For this review, take the finished solid that the model builds, in its own axes (mm). Face numbers are marked on the shaded views. Coordinates: 2 decimals unless noted, no trailing zeros. Order: outer loops, then holes, each group sorted by start corner. A loop starts at its lowest first (then second) coordinate and runs counter-clockwise, first axis right, second up. Notation, with made-up numbers: (56.25, 40.5) -> (115.25, 40.5) arc R23 cw to (115.25, 52.5) -> close; hole circle Ø2 at (-34.5, 1.25). An arc over 180 degrees is marked (long way). Answer as a JSON object with one key per item and string values. Group by question number.
1) Draft analysis for pull direction X (two halves, no side actions). For the marked faces 1, 2 and 3, state which applies: +X half, -X half, draft (parallel to the pull), parting line (faces both ways), or undercut.
2) Add section B-B, the plane x = 0. Write out the cut boundary in (y, z).
3) For pin 1 (8 mm diameter, centred on x = 5.5, y = 17.5, fed in from +Z); pin 2 (1 mm diameter, centred on y = 14.5, z = -10.5, fed in from +X); pin 3 (1 mm diameter, centred on y = 7, z = 10, fed in from +X); pin 4 (10 mm diameter, centred on x = 9, z = 10, fed in from +Y), all flat-tipped, find the tip position at first contact; note any pin that passes through.
4) Add section A-A, the plane z = 0. Write out the cut boundary in (x, y).
5) Add section C-C, the plane y = 13.25. Write out the cut boundary in (x, z), then the cut area to 3 significant figures.
6) Wall thickness on L1, parallel to X at y = 13.25, z = 0; L2, parallel to Y at x = 6.5, z = -6; L3, parallel to X at y = 8.5, z = -6.5: over which ranges is each line inside the solid? List them lowest first.
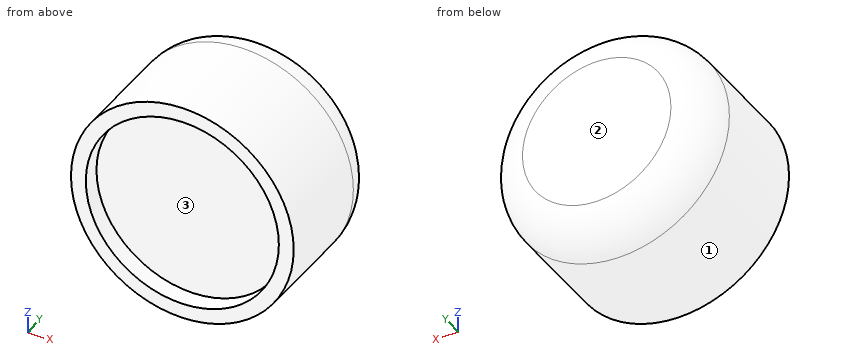
from build123d import *


with BuildPart() as part:
    # ｽｹｯﾁ1 → 回転1 (revolve)
    with BuildSketch(Plane.XY, mode=Mode.PRIVATE) as revolve_1_sk:
        with BuildLine():
            Line((0, 20), (10, 20))
            ThreePointArc((10, 20), (13.535533906, 18.535533906), (15, 15))
            Line((15, 15), (15, 1))
            Line((15, 1), (13, 1))
            Line((13, 1), (13, 3.5))
            Line((13, 3.5), (0, 3.5))
            Line((0, 3.5), (0, 6.5))
            Line((0, 6.5), (13, 6.5))
            Line((13, 6.5), (13, 15))
            ThreePointArc((13, 15), (12.121320344, 17.121320344), (10, 18))
            Line((10, 18), (0, 18))
            Line((0, 18), (0, 20))
        make_face()
    revolve(revolve_1_sk.sketch.rotate(Axis((0, 3.5, 0), (0, 1, 0)), 90), axis=Axis((0, 3.5, 0), (0, 1, 0)))


solid = part.part
Output values:
{
 "1": {"face 1": "parting line", "face 2": "draft", "face 3": "undercut"},
 "2": {"outline": "(1, -15) -> (15, -15) arc R5 ccw to (20, -10) -> (20, 10) arc R5 ccw to (15, 15) -> (1, 15) -> (1, 13) -> (3.5, 13) -> (3.5, -13) -> (1, -13) -> close; hole (6.5, -13) -> (15, -13) arc R3 ccw to (18, -10) -> (18, 10) arc R3 ccw to (15, 13) -> (6.5, 13) -> close"},
 "3": {"pin 1": "stops at z = 14.84", "pin 2": "stops at x = 11.18", "pin 3": "stops at x = 11.61", "pin 4": "stops at y = 20"},
 "4": {"outline": "(-15, 1) -> (-13, 1) -> (-13, 3.5) -> (13, 3.5) -> (13, 1) -> (15, 1) -> (15, 15) arc R5 ccw to (10, 20) -> (-10, 20) arc R5 ccw to (-15, 15) -> close; hole (-13, 6.5) -> (13, 6.5) -> (13, 15) arc R3 ccw to (10, 18) -> (-10, 18) arc R3 ccw to (-13, 15) -> close"},
 "5": {"outline": "circle Ø30 at (0, 0); hole circle Ø26 at (0, 0)", "area": "176 mm²"},
 "6": {"L1": "x = -15 to -13, 13 to 15", "L2": "y = 3.5 to 6.5, 18 to 20", "L3": "x = -13.52 to -11.26, 11.26 to 13.52"}
}
